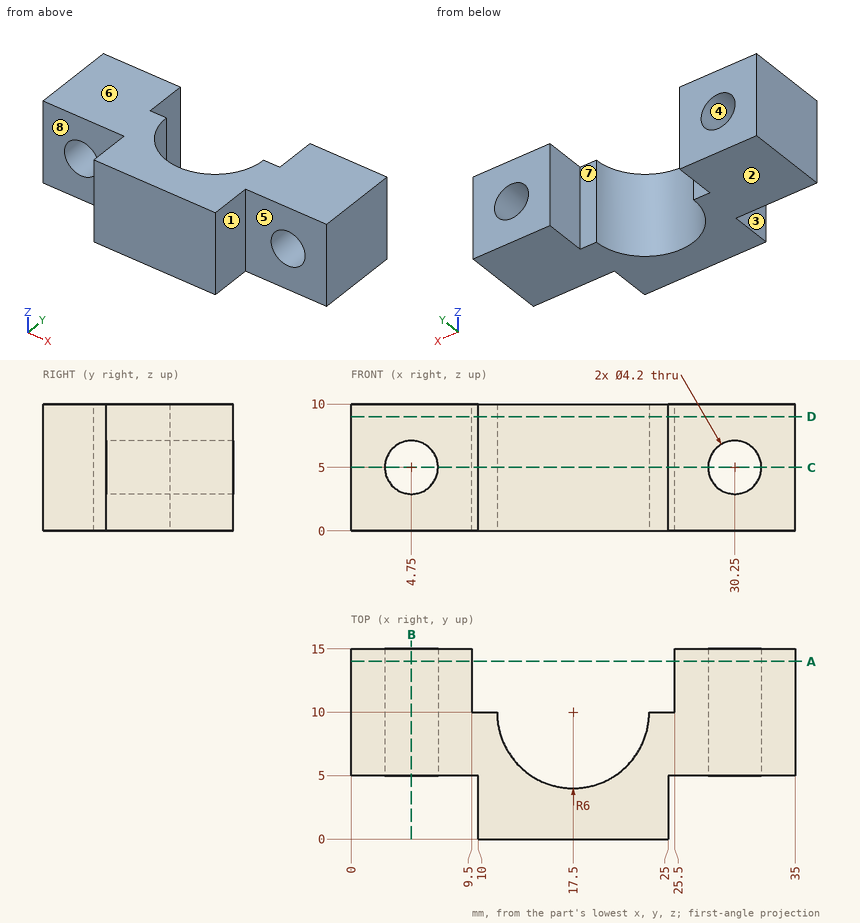
Verification items for this drawing (mm, ordinates from the low corner). A direction names the side the tool comes from. Give positions to 0.01 mm unless a question says otherwise; leave off trailing zeros. Loops run counter-clockwise (first coordinate to the right, second up) from the corner with the lowest first, then second, coordinate; pieces in that order, holes last. Notation, with made-up numbers: M -20.75,36.5 L 3.25,36.5 A12 cw 3.25,50.5 Z; hole C 70,53.5 d2. An arc over 180 degrees is marked long. Return JSON: item names as keys, results as strings. Group by question number.
1. Mould release check, pull along X, two halves, no side actions. Record for the marked faces 1, 2, 3 and 4: released by +X, released by -X, zero draft, split by the parting line, or undercut.
2. Go/stop test with flat-tipped pins: pin 1 (2.5 mm diameter, centred on y = 3.5, z = 5.5, fed in from -X); pin 2 (1.5 mm diameter, centred on x = 19.5, z = 3.5, fed in from +Y); pin 3 (1 mm diameter, centred on x = 5, z = 7, fed in from -Y). Record where each tip stops, or that it passes through.
3. Cross-section at B-B on x = 4.75. Record the boundary of the cut face in (y, z).
4. Cross-section at D-D on z = 9. Record the boundary of the cut face in (x, y), plus the area to 3 significant figures.
5. Thickness scan on L1, parallel to X at y = 11.75, z = 5; L2, parallel to X at y = 9.75, z = 5; L3, parallel to X at y = 11.5, z = 1.25. Record the ranges inside material, lowest first.
6. Tool access check on the marked faces 5, 6, 7 and 8. Record the directions out of +Z, -Z, +X, -X, +Y, -Y that give a thin tool (end or side, any length) a straight path to the whole face; none if there is none.
7. Cross-section at A-A on y = 14. Record the boundary of the cut face in (x, z), plus the area to 3 significant figures.
8. Cross-section at C-C on z = 5. Record the boundary of the cut face in (x, y).
Return value:
{
 "1": {"face 1": "released by +X", "face 2": "zero draft", "face 3": "released by -X", "face 4": "undercut"},
 "2": {"pin 1": "x = 10", "pin 2": "y = 4.67", "pin 3": "y = 5"},
 "3": {"outline": "M 5,0 L 15,0 L 15,2.9 L 5,2.9 Z; M 5,7.1 L 15,7.1 L 15,10 L 5,10 Z"},
 "4": {"outline": "M 0,5 L 10,5 L 10,0 L 25,0 L 25,5 L 35,5 L 35,15 L 25.5,15 L 25.5,10 L 23.5,10 A6 cw 11.5,10 L 9.5,10 L 9.5,15 L 0,15 Z", "area": "288 mm^2"},
 "5": {"L1": "0 to 2.65, 6.85 to 9.5, 25.5 to 28.15, 32.35 to 35", "L2": "0 to 2.65, 6.85 to 11.51, 23.49 to 28.15, 32.35 to 35", "L3": "0 to 9.5, 25.5 to 35"},
 "6": {"face 5": "+Z, -Z, +X, -Y", "face 6": "+Z, +X, -X, +Y, -Y", "face 7": "+Z, -Z, +Y", "face 8": "+Z, -Z, -X, -Y"},
 "7": {"outline": "M 0,0 L 9.5,0 L 9.5,10 L 0,10 Z; M 25.5,0 L 35,0 L 35,10 L 25.5,10 Z; hole C 4.75,5 d4.2; hole C 30.25,5 d4.2", "area": "162 mm^2"},
 "8": {"outline": "M 0,5 L 2.65,5 L 2.65,15 L 0,15 Z; M 6.85,5 L 10,5 L 10,0 L 25,0 L 25,5 L 28.15,5 L 28.15,15 L 25.5,15 L 25.5,10 L 23.5,10 A6 cw 11.5,10 L 9.5,10 L 9.5,15 L 6.85,15 Z; M 32.35,5 L 35,5 L 35,15 L 32.35,15 Z"}
}
